```python
from build123d import *

# Parameters (mm, degrees)
F0_W     = 63.5
F0_H     = 44.45
F1_DEPTH = 63.5
F2_START = 58.674
F2_DEPTH = 4.826
F3_SIZE  = 5.08


with BuildPart() as f1:
    # F0 (on Front) → F1 (new body)
    with BuildSketch(Plane.XZ):
        Polygon((-48.8091893494, -44.45), (-31.75, -44.45), (-31.75, 0), align=None)
        with Locations((0, -22.225)):
            Rectangle(F0_W, F0_H)
        Polygon((31.75, 0), (31.75, -44.45), (48.8091893494, -44.45), align=None)
    extrude(amount=F1_DEPTH)

    # F0 (on Front) → F2 (join)
    with BuildSketch(Plane.XZ.offset(F2_START)):
        with Locations((0, 22.225)):
            Rectangle(F0_W, F0_H)
    extrude(amount=F2_DEPTH)

    # F3
    f3_edges = [f1.edges().sort_by_distance(p)[0] for p in [
        (0, -58.674, 0),
    ]]
    chamfer(f3_edges, length=F3_SIZE)


solid = f1.part
```
Could you check a few things on this model? Use its own coordinates, in mm. A direction names the side the tool comes from. Coordinates: 2 decimals unless noted, no trailing zeros. Order: outer loops, then holes, each group sorted by start corner. A loop starts at its lowest first (then second) coordinate and runs counter-clockwise, first axis right, second up. Notation, with made-up numbers: M -33,66 L -10,66 A27 cw -10,95 Z; hole C -7.75,86 d5. An arc over 180 degrees is marked long. Use one line per item in the form item = value. Start each with the question number.
1. For pin 1 (3 mm diameter, centred on y = -43.5, z = -7, fed in from +X); pin 2 (3 mm diameter, centred on y = -56, z = 13.5, fed in from +X); pin 3 (8 mm diameter, centred on y = -57.5, z = 25.5, fed in from -X); pin 4 (5 mm diameter, centred on y = -21.5, z = 0, fed in from -X), each with a flat end and sliding along its axis, tell me the tip position at first contact or that it passes through.
2. Suppose I cut it at C-C on y = -51. Write out the boundary of the cut face in (x, z).
3. Please list where these lines run through material, in increasing order: line 1 (Z direction, x = -20.5, y = -53.5); line 2 (Y direction, x = 31.5, z = 37.5); line 3 (X direction, y = -22, z = -10).
4. On a 3-axis mill with a long thin cutter (end or side, diameter ignored), from which of +Z, -Z, +X, -X, +Y, -Y can I reach the whole of each face in a straight line? I mean faces 1 (the flat face through (0, -26, 0)), 2 (the flat face through (31.75, -61, 22)), 3 (the flat face through (-31.75, -61, 22)). Say none if no direction works.
5. We'd pull the mould along Z, two halves only. Please class faces 4 (the flat face through (-0.444, -56.098, 2.504)), 5 (the flat face through (-1, -31, -44.45)), 6 (the flat face through (-1, -63.5, -9)): +Z half, -Z half, draft (parallel to the pull), parting line (faces both ways), or undercut.
6. Suppose I cut it at B-B on z = 15.5. Write out the boundary of the cut face in (x, y).
7. Suppose I cut it at A-A on x = -29.5. Write out the boundary of the cut face in (y, z), then the cut area to 3 significant figures.
Geometry says:
q1.pin_1 = 35.01
q1.pin_2 = through
q1.pin_3 = -31.75
q1.pin_4 = -32.71
q2.outline = M -48.81,-44.45 L 48.81,-44.45 L 31.75,0 L -31.75,0 Z
q3.line_1 = -44.45 to 0
q3.line_2 = -63.5 to -58.67
q3.line_3 = -35.59 to 35.59
q4.face_1 = +Z, +X, -X, +Y
q4.face_2 = +Z, +X, +Y, -Y
q4.face_3 = +Z, -X, +Y, -Y
q5.face_4 = +Z half
q5.face_5 = -Z half
q5.face_6 = draft
q6.outline = M -31.75,-63.5 L 31.75,-63.5 L 31.75,-58.67 L -31.75,-58.67 Z
q7.outline = M -63.5,-44.45 L 0,-44.45 L 0,0 L -53.59,0 L -58.67,5.08 L -58.67,44.45 L -63.5,44.45 Z
q7.area = 3,050 mm^2
